Source: CAD feature listing. Evaluate the final solid. Frame: model axes, mm. Face numbers are marked on the shaded views. A direction names the side the tool comes from. Coordinates: 2 decimals unless noted, no trailing zeros. Loops run counter-clockwise (first coordinate to the right, second up) from the corner with the lowest first, then second, coordinate; pieces in that order, holes last.
Item 1: Section query B-B, the plane z = 25.95. Return the cut outline in (x, y), then the cut area to 3 significant figures.
Item 2: Section query C-C, the plane y = -2. Return the cut outline in (x, z), then the cut area to 3 significant figures.
Item 3: Reachability of the marked faces 1 and 2 from +Z, -Z, +X, -X, +Y, -Y: full face, straight path, thin tool, end or side. Return the list, or none.
Item 4: Line query: probe 1 along Y at (x, z) = (-11.45, 25.8); probe 2 along Y at (x, z) = (-9.65, 25.75); probe 3 along Z at (x, y) = (-11.4, -1.25). Output: solid intervals per line, ascending.
```python
from build123d import *

# Parameters (mm, degrees)
F0_W     = 4.35
F0_H     = 1.8
F1_DEPTH = 11.7
F2_R     = 1.84
F3_DEPTH = 5.1
F5_DEPTH = 25
F6_W     = 5.1
F6_H     = 0.197361
F7_DEPTH = 25


with BuildPart() as f1:
    # F0 (on Front) → F1 (new body)
    with BuildSketch(Plane.XZ):
        with Locations((-12.080966, 25.862558)):
            Rectangle(F0_W, F0_H)
    extrude(amount=F1_DEPTH)

    # F2 (on face) → F3 (join)
    with BuildSketch(Plane(origin=(-14.255966, 0, 0), x_dir=(0, -1, 0), z_dir=(-1, 0, 0))):
        with Locations((11.043573, 25.862558)):
            Circle(F2_R)
    extrude(amount=-F3_DEPTH)

    # F4 (on face) → F5 (cut)
    with BuildSketch(Plane(origin=(-14.255966, 0, 0), x_dir=(0, -1, 0), z_dir=(-1, 0, 0))):
        Polygon((10.555248, 28.524822), (9.438705, 26.762558), (31.722508, 26.762558), align=None)
    extrude(amount=-F5_DEPTH, mode=Mode.SUBTRACT)

    # F6 (on face) → F7 (cut)
    with BuildSketch(Plane(origin=(0, 5.36427, 3.39872), x_dir=(1, 0, 0), z_dir=(0, -0.844723, -0.535204))):
        with Locations((-11.705966, 27.757259)):
            Rectangle(F6_W, F6_H)
    extrude(amount=-F7_DEPTH, mode=Mode.SUBTRACT)


solid = f1.part
```
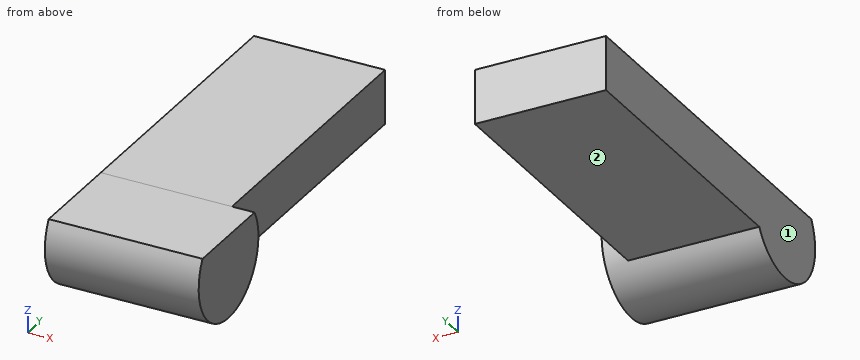
Verdict:
1. outline: (-14.26, -12.88) - (-9.16, -12.88) - (-9.16, -9.21) - (-9.91, -9.21) - (-9.91, 0) - (-14.26, 0) - close
1. area: 58.8 mm2
2. outline: (-14.26, 24.96) - (-9.91, 24.96) - (-9.91, 26.76) - (-14.26, 26.76) - close
2. area: 7.83 mm2
3. face 1: +Z, -Z, -X, +Y, -Y
3. face 2: -Z, +X, -X, +Y
4. probe 1: y = -12.88 to 0
4. probe 2: y = -12.88 to -9.21
4. probe 3: z = 24.96 to 26.76
